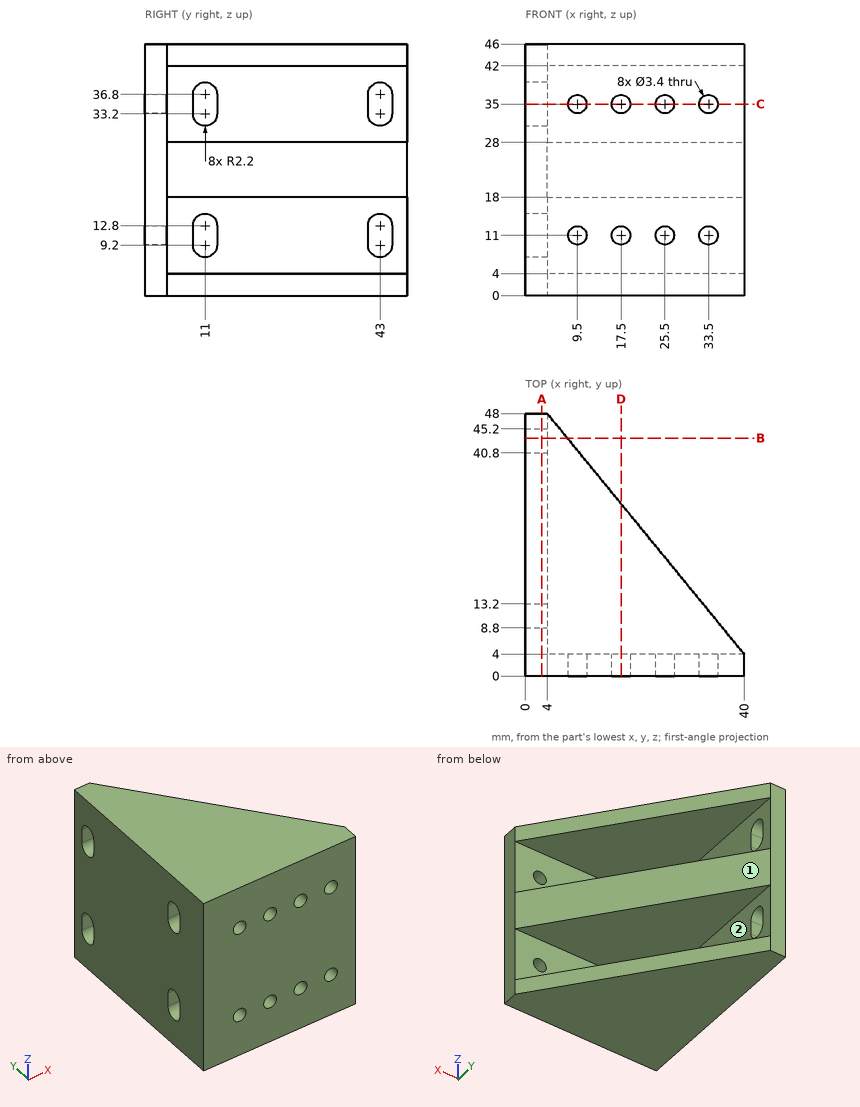
Geometry: see drawing. Coordinates: mm, zero at the bounding-box minimum. A direction names the side the tool comes from. Round coordinates to 2 decimals unless told otherwise and drop trailing zeros. Write each loop counter-clockwise with the first axis right and the second up, starting at its lowest first coordinate (ties: lowest second). Pieces come first, ordered by that corner, then holes.
Item 1: Section query C-C (z = 35). Give the number of separate pieces and of enclosed holes in the cut face, plus the area to 3 significant figures.
Item 2: Section query B-B (y = 43.5). Return loops of the section in (x, z), plus the area to 3 significant figures.
Item 3: Material intervals for L1, parallel to Z at x = 5, y = 34.5; L2, parallel to Z at x = 9.5, y = 2.85; L3, parallel to X at y = 21, z = 17.5, sorted ascending.
Item 4: Pin query (flat end, axial travel): P1, Ø3, axis at y = 23.5, z = 15, coming from the +X side; P2, Ø4, axis at x = 9.5, z = 35, coming from the +Y side; P3, Ø15.5, axis at x = 19.5, z = 12.5, coming from the +Y side. Return the tip coordinate at first contact, or that it passes through.
Item 5: Section query D-D (x = 17.5). Return loops of the section in (y, z), plus the area to 3 significant figures.
Item 6: Section query A-A (x = 3). Return loops of the section in (y, z).
Item 7: Set-up query: the marked faces 1 and 2. Return all of +Z, -Z, +X, -X, +Y, -Y with unobstructed straight access to the full face (end or side cutting, diameter ignored); none if empty.
Completed:
1. separate pieces: 7
1. enclosed holes: 0
1. area: 246 mm2
2. outline: (0, 0) - (7.68, 0) - (7.68, 4) - (4, 4) - (4, 7.06) - (0, 7.06) - close; (0, 14.94) - (4, 14.94) - (4, 18) - (7.68, 18) - (7.68, 28) - (4, 28) - (4, 31.06) - (0, 31.06) - close; (0, 38.94) - (4, 38.94) - (4, 42) - (7.68, 42) - (7.68, 46) - (0, 46) - close
2. area: 187 mm2
3. L1: z = 0 to 4, 18 to 28, 42 to 46
3. L2: z = 0 to 9.3, 12.7 to 33.3, 36.7 to 46
3. L3: x = 0 to 4
4. P1: stops at x = 4
4. P2: stops at y = 4
4. P3: stops at y = 35.73
5. outline: (0, 0) - (31.5, 0) - (31.5, 4) - (4, 4) - (4, 9.3) - (0, 9.3) - close; (0, 12.7) - (4, 12.7) - (4, 18) - (31.5, 18) - (31.5, 28) - (4, 28) - (4, 33.3) - (0, 33.3) - close; (0, 36.7) - (4, 36.7) - (4, 42) - (31.5, 42) - (31.5, 46) - (0, 46) - close
5. area: 652 mm2
6. outline: (0, 0) - (48, 0) - (48, 46) - (0, 46) - close; hole (8.8, 9.2) arc R2.2 ccw to (13.2, 9.2) - (13.2, 12.8) arc R2.2 ccw to (8.8, 12.8) - close; hole (8.8, 33.2) arc R2.2 ccw to (13.2, 33.2) - (13.2, 36.8) arc R2.2 ccw to (8.8, 36.8) - close; hole (40.8, 9.2) arc R2.2 ccw to (45.2, 9.2) - (45.2, 12.8) arc R2.2 ccw to (40.8, 12.8) - close; hole (40.8, 33.2) arc R2.2 ccw to (45.2, 33.2) - (45.2, 36.8) arc R2.2 ccw to (40.8, 36.8) - close
7. face 1: +Z, -Z, +X, +Y
7. face 2: +X, +Y
